```python
from build123d import *

# Parameters (mm, degrees)
BOSS_EXTRUDE1_DEPTH = 19.05


with BuildPart() as part:
    # Sketch1 → Boss-Extrude1 (new body)
    with BuildSketch(Plane(origin=(0, 0, 0), x_dir=(1, 0, 0), z_dir=(0, 1, 0))):
        with BuildLine():
            Line((0, 0), (-50.8, 0))
            ThreePointArc((-50.8, 0), (-58.469137427, 3.673291188), (-60.413921301, 11.951367819))
            Line((-60.413921301, 11.951367819), (-19.05, 200.52150033))
            ThreePointArc((-19.05, 200.52150033), (-22.940110947, 273.310750301), (-63.619044117, 333.79737916))
            ThreePointArc((-63.619044117, 333.79737916), (-75.370955214, 343.219242923), (-87.729421071, 351.830122835))
            ThreePointArc((-87.729421071, 351.830122835), (-90.543698917, 365.003242823), (-77.370578929, 367.817520668))
            ThreePointArc((-77.370578929, 367.817520668), (-53.490221725, 350.184763018), (-31.937222332, 329.772663182))
            ThreePointArc((-31.937222332, 329.772663182), (5.842491744, 269.993724887), (19.05, 200.52150033))
            Line((19.05, 200.52150033), (0, 200.52150033))
            Line((0, 200.52150033), (0, 0))
        make_face()
    extrude(amount=BOSS_EXTRUDE1_DEPTH)


solid = part.part
```
The listing builds one solid part. Answer for the finished solid, in the listing's coordinates (mm). A direction names the side the tool comes from. Coordinates: 2 decimals unless noted, no trailing zeros. Write each loop counter-clockwise with the first axis right and the second up, starting at its lowest first coordinate (ties: lowest second). Pieces come first, ordered by that corner, then holes. Notation, with made-up numbers: (38, -5.75) - (45, -5.75) arc R9 cw to (45, 3.25) - close; hole circle Ø9 at (6.25, 70.25). An arc over 180 degrees is marked (long way). Return JSON: item names as keys, results as strings. Group by question number.
Q1. For a pull along Z with two mould halves and no side action, classify faces 1 (the flat face through (-25, 9, 0)), 2 (the flat face through (0, 9, -102)), 3 (the cylindrical face through (-22.616, 9.392, -272.33)), 4 (the cylindrical face through (-90.656, 9.392, -364.826)) as +Z half, -Z half, draft (parallel to the pull), parting line (faces both ways), or undercut.
Q2. Flat-ended cylindrical pins translate along their axes: pin 1 Ø5.5 at (x, y) = (9, 12) entering from +Z; pin 2 Ø4 at (y, z) = (3, -135.5) entering from -X; pin 3 Ø3 at (y, z) = (3, -52.5) entering from -X; pin 4 Ø3 at (x, z) = (-21.5, -205.5) entering from +Y. Find the tip coordinate at first contact, or state that the pin passes through.
Q3. Which of the six approach directions +Z, -Z, +X, -X, +Y, -Y give full straight-line access (tool end or side, diameter ignored) to faces 5 (the cylindrical face through (5.475, 9.392, -270.919)), 6 (the flat face through (10, 9, -200.522)), 7 (the flat face through (-40.02, 9.39, -104.92))?
Q4. Find the intervals of material crossed by line 1 along X through (y, z) = (17, -98.5); line 2 along X through (y, z) = (15, -316); line 3 along Z through (x, y) = (-82, 8.25), in increasing order. Write a range as [from, to].
Q5. The part is cut by section C-C on x = -82.55. Write down the section's boundary in (y, z), and give its area (3 significant figures).
Q6. The part is cut by section B-B on z = -233.5. Write down the section's boundary in (x, y).
Evaluation:
{
 "1": {"face 1": "+Z half", "face 2": "draft", "face 3": "undercut", "face 4": "parting line"},
 "2": {"pin 1": "stops at z = -200.52", "pin 2": "stops at x = -33.75", "pin 3": "stops at x = -51.85", "pin 4": "passes through"},
 "3": {"face 5": "-Z, +X, +Y, -Y", "face 6": "+Z, +X, +Y, -Y", "face 7": "-X, +Y, -Y"},
 "4": {"line 1": "x = [-41.43, 0]", "line 2": "x = [-46.34, -20.25]", "line 3": "z = [-369.33, -347.99]"},
 "5": {"outline": "(0, -369.35) - (19.05, -369.35) - (19.05, -348.37) - (0, -348.37) - close", "area": "400 mm2"},
 "6": {"outline": "(-15.92, 0) - (16.16, 0) - (16.16, 19.05) - (-15.92, 19.05) - close"}
}
